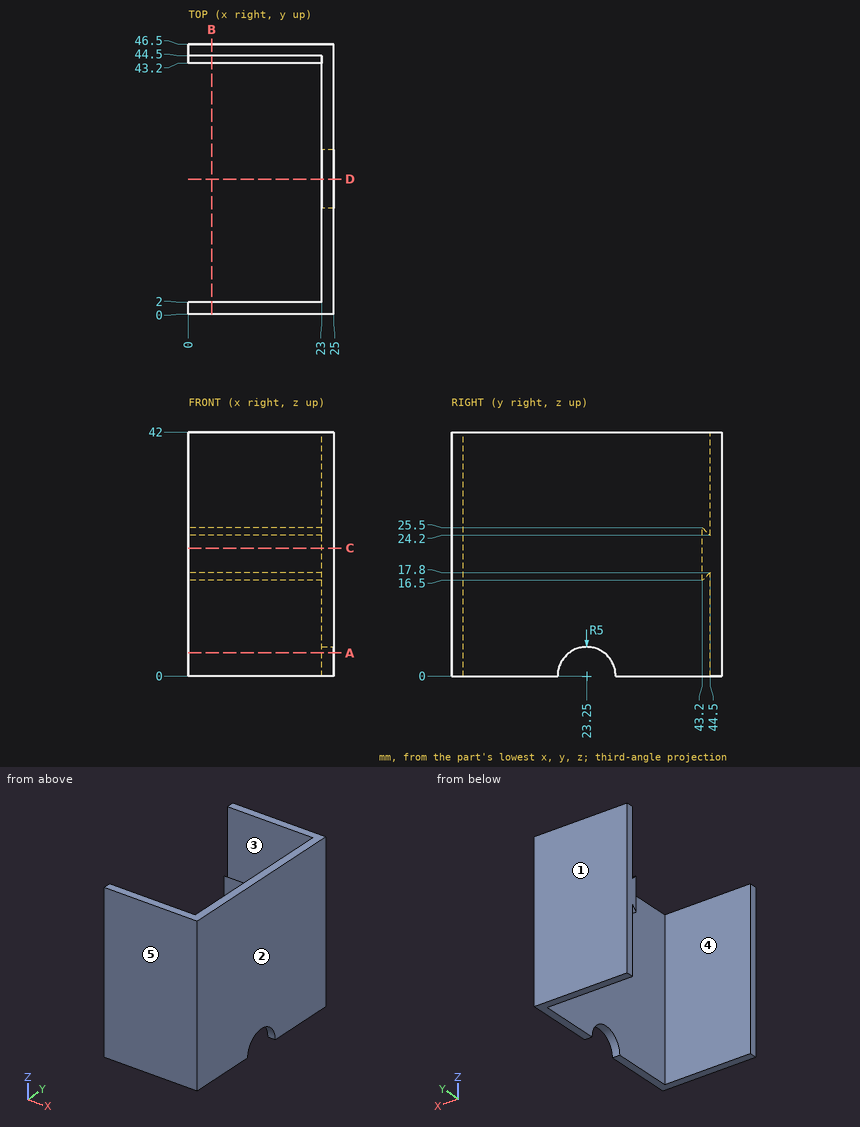
Could you check a few things on this drawing? It's one solid part, dimensions in mm from its lowest x, y, z. A direction names the side the tool comes from. Coordinates: 2 decimals unless noted, no trailing zeros. Order: outer loops, then holes, each group sorted by start corner. A loop starts at its lowest first (then second) coordinate and runs counter-clockwise, first axis right, second up. Notation, with made-up numbers: (62.5, 24) - (91.5, 24) arc R13 cw to (91.5, 43) - close; hole circle Ø7 at (16.5, -17.5). An arc over 180 degrees is marked (long way). One line per question, with ' | ' between items. Start each with the question number.
1. If we mould it in two halves opening along Y, with no side actions, what happens to the marked faces 1, 2 and 3? For each: released by +Y, released by -Y, zero draft, split by the parting line, or undercut.
2. I'm going to push flat-ended pins straight in: pin 1 Ø3 at (y, z) = (19, 19.5) entering from -X; pin 2 Ø2.5 at (x, z) = (13, 19) entering from -Y. Where does each tip first touch, or does it pass through?
3. Please list where these lines run through material, in increasing order: line 1 along Y through (x, z) = (4.25, 16); line 2 along X through (y, z) = (21, 15); line 3 along Y through (x, z) = (8.25, 23.5). Write a range as [from, to].
4. If we section it at D-D (y = 23.25): Write out the boundary of the cut face in (x, z), and give its area (3 significant figures).
5. If we section it at B-B (x = 4): Write out the boundary of the cut face in (y, z).
6. Which directions (+Z, -Z, +X, -X, +Y, -Y) give clear straight access to the entire face, cutting with the end or side of a thin tool? Please do the marked faces 4 and 5.
7. If we section it at A-A (z = 4): Write out the boundary of the cut face in (x, y).
8. If we section it at C-C (z = 22): Write out the boundary of the cut face in (x, y), and give its area (3 significant figures).
Model answer:
1) face 1: released by +Y | face 2: zero draft | face 3: undercut
2) pin 1: stops at x = 23 | pin 2: stops at y = 0
3) line 1: y = [0, 2], [44.5, 46.5] | line 2: x = [23, 25] | line 3: y = [0, 2], [43.2, 46.5]
4) outline: (23, 5) - (25, 5) - (25, 42) - (23, 42) - close | area: 74.0 mm²
5) outline: (0, 0) - (2, 0) - (2, 42) - (0, 42) - close; (43.2, 16.5) - (44.5, 17.8) - (44.5, 0) - (46.5, 0) - (46.5, 42) - (44.5, 42) - (44.5, 24.2) - (43.2, 25.5) - close
6) face 4: +Z, -Z, -X | face 5: +Z, -Z, +X, -X, -Y
7) outline: (0, 0) - (25, 0) - (25, 20.25) - (23, 20.25) - (23, 2) - (0, 2) - close; (0, 44.5) - (23, 44.5) - (23, 26.25) - (25, 26.25) - (25, 46.5) - (0, 46.5) - close
8) outline: (0, 0) - (25, 0) - (25, 46.5) - (0, 46.5) - (0, 43.2) - (23, 43.2) - (23, 2) - (0, 2) - close | area: 215 mm²
